Job drawing, mm, ordinate dimensions from the low corner. One solid piece. Coordinates: 2 decimals unless noted, no trailing zeros. Write each loop counter-clockwise with the first axis right and the second up, starting at its lowest first coordinate (ties: lowest second). Pieces come first, ordered by that corner, then holes. Notation, with made-up numbers: (49.25, 39.5) -> (86.25, 39.5) arc R32 cw to (86.25, 72.5) -> close; hole circle Ø2 at (75, 3). An arc over 180 degrees is marked (long way). One line per question, with ' | ' between items. Start each with the question number.
Item 1: Two-plate mould, pull along X, no slides. Class the marked faces 1, 2 and 3: pulls with the +X half, pulls with the -X half, needs draft (parallel to the pull), parting line crosses it, or undercut.
Item 2: Pin check, flat tips, straight feed: pin 1 (8 mm diameter, centred on x = 70, z = 49, fed in from -Y); pin 2 (8 mm diameter, centred on x = 33.5, z = 73, fed in from +Y); pin 3 (3 mm diameter, centred on x = 71, z = 75, fed in from -Y). Stop position of each tip, or through.
Item 3: Saw through at C-C (z = 37). List the corners of the cut face in (x, y).
Item 4: Saw through at B-B (z = 69). List the corners of the cut face in (x, y).
Item 5: Probe probe 1 along Y at (x, z) = (55, 70); probe 2 along X at (y, z) = (56.5, 22.5); probe 3 along Y at (x, z) = (55, 17). List the from-to ranges inside material, lowest first. Write a range as [from, to].
Item 6: Saw through at A-A (x = 55). List the corners of the cut face in (y, z), and give its area (3 significant figures).
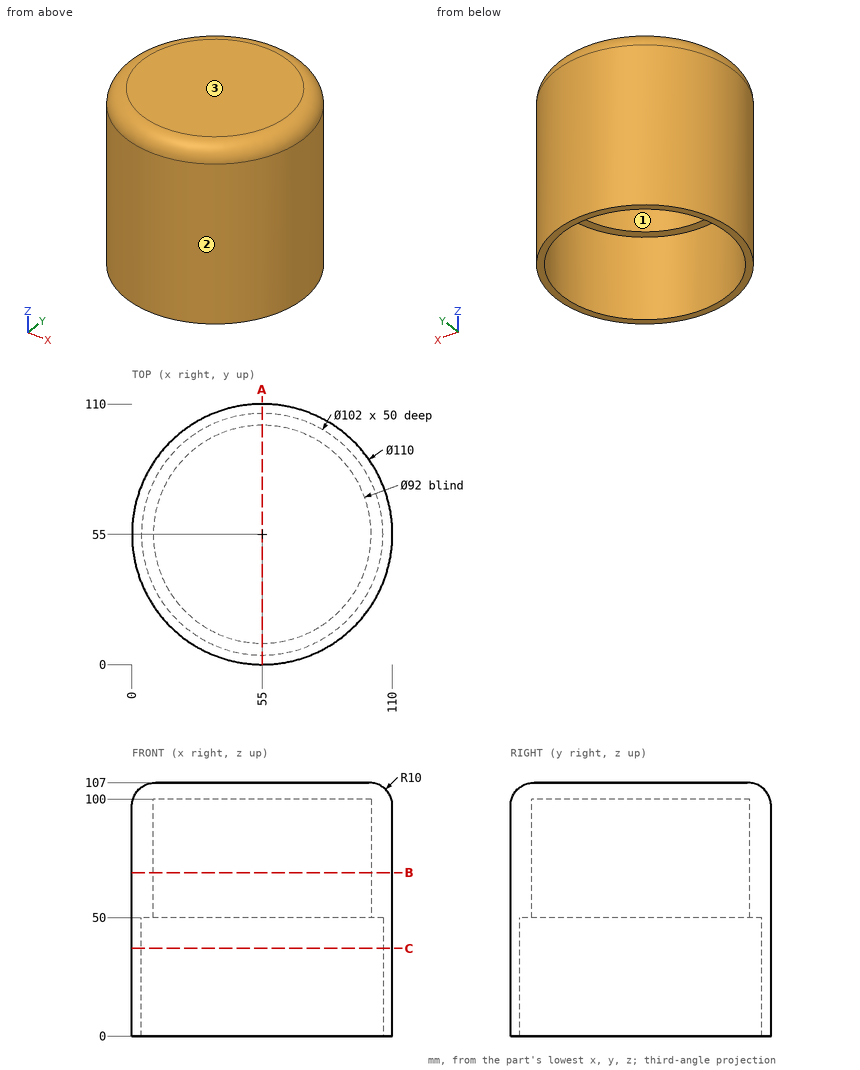
From the geometry:
1) face 1: undercut | face 2: parting line crosses it | face 3: needs draft
2) pin 1: y = 1.11 | pin 2: y = 107.14 | pin 3: y = 1.95
3) outline: circle Ø110 at (55, 55); hole circle Ø102 at (55, 55)
4) outline: circle Ø110 at (55, 55); hole circle Ø92 at (55, 55)
5) probe 1: [0, 9], [101, 110] | probe 2: [0.02, 4.02], [105.98, 109.98] | probe 3: [0, 4], [106, 110]
6) outline: (0, 0) -> (4, 0) -> (4, 50) -> (9, 50) -> (9, 100) -> (101, 100) -> (101, 50) -> (106, 50) -> (106, 0) -> (110, 0) -> (110, 97) arc R10 ccw to (100, 107) -> (10, 107) arc R10 ccw to (0, 97) -> close | area: 2,030 mm2
